```python
from build123d import *

# Parameters (mm, degrees)
F2_R     = 3.75
F3_DEPTH = 1.2
F4_R     = 2.5
F5_DEPTH = 4.5
F6_R     = 1.55
F7_DEPTH = 4.5
F8_SIZE2 = 0.5
F8_SIZE  = 0.5


with BuildPart() as f1:
    # F0 (on Front) → F1 (revolve)
    with BuildSketch(Plane.XZ):
        with BuildLine():
            Line((-8.5, 0), (0, 0))
            Line((0, 0), (0, 0.346079265))
            add(Edge.make_bspline(
                [(-8.5, 1), (-7.9439580441, 0.9699382936), (-6.4414965177, 1.1872948826), (-4.7760567404, 0.3213823797), (-1.4301329999, 0.5005030041), (-0.8624908504, 0.3459224587), (0, 0.346079265)],
                knots=[0, 0, 0, 0, 0.2391975808, 0.4806677273, 0.7782536308, 1, 1, 1, 1], degree=3))
            Line((-8.5, 1), (-8.5, 0))
        make_face()
    revolve(axis=Axis((0, 0, 0.599608873), (0, 0, 1)))

    # F2 (on face) → F3 (join)
    with BuildSketch(Plane(origin=(0, 0, 0), x_dir=(1, 0, 0), z_dir=(0, 0, -1))):
        Circle(F2_R)
    extrude(amount=F3_DEPTH)

    # F4 (on face) → F5 (join)
    with BuildSketch(Plane(origin=(0, 0, -1.2), x_dir=(1, 0, 0), z_dir=(0, 0, -1))):
        Circle(F4_R)
    extrude(amount=F5_DEPTH)

    # F6 (on face) → F7 (cut, through all)
    with BuildSketch(Plane(origin=(0, 0, -5.7), x_dir=(1, 0, 0), z_dir=(0, 0, -1))):
        Circle(F6_R)
    extrude(amount=-F7_DEPTH, mode=Mode.SUBTRACT)

    # F8
    f8_edges = [f1.edges().sort_by_distance(p)[0] for p in [
        (-3.75, 0, -1.2),
        (8.5, 0, 0),
    ]]
    chamfer(f8_edges, length=F8_SIZE, length2=F8_SIZE2)


solid = f1.part
```
Input: part model. Units: mm. Frame: model coordinates. A direction names the side the tool comes from. Give positions to 0.01 mm unless a question says otherwise; leave off trailing zeros. Order: outer loops, then holes, each group sorted by start corner. A loop starts at its lowest first (then second) coordinate and runs counter-clockwise, first axis right, second up.
1. Material intervals for L1, parallel to X at y = 0, z = -3; L2, parallel to Z at x = -7.25, y = 0.75, sorted ascending.
Derived:
L1: x = -2.5 to -1.55, 1.55 to 2.5
L2: z = 0 to 1.03
2. Section B-B on z = -2. Return the cut outline in (x, y), and give its area (3 significant figures).
Derived:
outline: circle Ø5 at (0, 0); hole circle Ø3.1 at (0, 0)
area: 12.1 mm2
3. Pin query (flat end, axial travel): pin 1 (1.6 mm diameter, centred on x = 0, y = 0, fed in from -Z); pin 2 (8 mm diameter, centred on x = -3.5, y = -1.5, fed in from -Z); pin 3 (1.5 mm diameter, centred on y = 2.5, z = -0.5, fed in from +X); pin 4 (1.9 mm diameter, centred on x = 0, y = 0, fed in from +Z). Return the tip coordinate at first contact, or that it passes through.
Derived:
pin 1: stops at z = -1.2
pin 2: stops at z = -5.7
pin 3: stops at x = 7.89
pin 4: stops at z = 0.38
4. Reachability of faces 4 (the cylindrical face through (-0.54, 2.44, -3.42)), 5 (the cylindrical face through (-4.57, -7.167, 0.746)) from +Z, -Z, +X, -X, +Y, -Y: full face, straight path, thin tool, end or side. Return the list, or none.
Derived:
face 4: -Z
face 5: +Z, -Z
5. Mould query, pull axis X, two halves, no side actions, for faces 1 (the flat face through (0, 2, -5.7)), 2 (the cylindrical face through (-3.746, -0.165, -0.345)), 3 (the flat face through (0, 0, -1.2)). Classes: released by +X, released by -X, zero draft, split by the parting line, or undercut.
Derived:
face 1: zero draft
face 2: split by the parting line
face 3: undercut
6. Section A-A on z = -0.5. Return the cut outline in (x, y).
Derived:
outline: circle Ø7.5 at (0, 0)
